from build123d import *

# Parameters (mm, degrees)
F0_R      = 55
F1_DEPTH  = 3.6
F2_R      = 44.5
F3_DEPTH  = 2.7
F4_R      = 37.5
F5_DEPTH  = 0.8
F6_R      = 17.5
F7_DEPTH  = 15
F8_SIZE   = 2
F10_D     = 20
F10_DEPTH = 13
F10_TIP   = 6.0086061903
F13_D     = 13.5
F14_SIZE  = 1
F15_SIZE  = 1


with BuildPart() as f1:
    # F0 (on Top) → F1 (new body)
    with BuildSketch(Plane.XY):
        Circle(F0_R)
    extrude(amount=-F1_DEPTH)

    # F2 (on face) → F3 (join)
    with BuildSketch(Plane(origin=(0, 0, -3.6), x_dir=(1, 0, 0), z_dir=(0, 0, -1))):
        Circle(F2_R)
    extrude(amount=F3_DEPTH)

    # F4 (on face) → F5 (join)
    with BuildSketch(Plane(origin=(0, 0, -6.3), x_dir=(1, 0, 0), z_dir=(0, 0, -1))):
        Circle(F4_R)
    extrude(amount=F5_DEPTH)

    # F6 (on face) → F7 (join)
    with BuildSketch(Plane(origin=(0, 0, -7.1), x_dir=(1, 0, 0), z_dir=(0, 0, -1))):
        Circle(F6_R)
    extrude(amount=F7_DEPTH)

    # F8
    f8_edges = [f1.edges().sort_by_distance(p)[0] for p in [
        (-17.5, 0, -22.1),
    ]]
    chamfer(f8_edges, length=F8_SIZE)

    # F10
    with Locations(Plane.XY):
        with Locations((0, 0)):
            Hole(F10_D / 2, depth=F10_DEPTH)
            with Locations((0, 0, -(F10_DEPTH + F10_TIP / 2))):  # 118° drill point
                Cone(0, F10_D / 2, F10_TIP, mode=Mode.SUBTRACT)

    # F13 (through all)
    with Locations(Plane(origin=(0, 0, -22.1), x_dir=(1, 0, 0), z_dir=(0, 0, -1))):
        with Locations((0, 0)):
            Hole(F13_D / 2)

    # F14
    f14_edges = [f1.edges().sort_by_distance(p)[0] for p in [
        (-55, 0, 0),
    ]]
    chamfer(f14_edges, length=F14_SIZE)

    # F15
    f15_edges = [f1.edges().sort_by_distance(p)[0] for p in [
        (-55, 0, -3.6),
    ]]
    chamfer(f15_edges, length=F15_SIZE)


solid = f1.part
Build history of the part. All positions in model axes, mm. A direction names the side the tool comes from. Round coordinates to 2 decimals unless told otherwise and drop trailing zeros. Order: outer loops, then holes, each group sorted by start corner. A loop starts at its lowest first (then second) coordinate and runs counter-clockwise, first axis right, second up. Notation, with made-up numbers: M 62.5,9.25 L 84.5,9.25 A22 ccw 84.5,43.25 Z; hole C 48.25,32 d3. An arc over 180 degrees is marked long. Use CSV: the item, a comma, the result in double quotes. Start each with the question number.
(1) Cut at D-D on z = -8.5. List the corners of the cut face in (x, y).
(2) Flat gauge pins, fed straight in: P1, Ø1.5, axis at x = -6, y = -43, coming from the -Z side; P2, Ø6, axis at x = 7, z = -16, coming from the -Y side; P3, Ø11, axis at x = 0, y = 0, coming from the +Z side (1 decimal); P4, Ø5, axis at y = 21.5, z = -2.5, coming from the +X side. Where does each tip first touch, or does it go through?
(3) Mould opens along Y. For faces 1 (the face through (8, 16, -7.1)), 2 (the face through (2.17, -9.76, -6.59)), 3 (the face through (-13.887, 10.648, -13.509)) say: +Y half, -Y half, draft (parallel to the pull), parting line (faces both ways), or undercut.
(4) Tool access for faces 4 (the face through (11, 1, 0)), 5 (the face through (-20, 33, -6.3)): list every direction of +Z, -Z, +X, -X, +Y, -Y with a clear straight run to the whole face (end or side of a thin tool).
(5) Drill centre lines: probe 1 along Y at (x, z) = (0, -10); probe 2 along Z at (x, y) = (-17.5, 15.5). Where is each one in solid material? Low to high.
(6) Cut at C-C on z = -17. List the corners of the cut face in (x, y), then the cut area to 3 significant figures.
Findings:
1,outline,"C 0,0 d35; hole C 0,0 d20"
2,P1,"stops at z = -6.3"
2,P2,"stops at y = -17.04"
2,P3,"passes through"
2,P4,"stops at x = 51.61"
3,face 1,"draft"
3,face 2,"undercut"
3,face 3,"parting line"
4,face 4,"+Z, +X, -X, +Y, -Y"
4,face 5,"-Z"
5,probe 1,"y = -17.5 to -10, 10 to 17.5"
5,probe 2,"z = -7.1 to 0"
6,outline,"C 0,0 d35; hole C 0,0 d13.5"
6,area,"819 mm^2"
